from build123d import *

# Parameters (mm, degrees)
SKETCH1_R           = 25.4
BOSS_EXTRUDE1_DEPTH = 10.16
FILLET1_R           = 0.762
CUT_EXTRUDE1_DEPTH  = 11.16


with BuildPart() as part:
    # Sketch1 → Boss-Extrude1 (new body)
    with BuildSketch(Plane(origin=(0, 0, 0), x_dir=(0, 0, -1), z_dir=(1, 0, 0))):
        Circle(SKETCH1_R)
    extrude(amount=BOSS_EXTRUDE1_DEPTH)

    # Fillet1
    fillet1_edges = [part.edges().sort_by_distance(p)[0] for p in [
        (0, 0, 25.4),
        (10.16, 0, 25.4),
    ]]
    fillet(fillet1_edges, radius=FILLET1_R)

    # Sketch2 → Cut-Extrude1 (cut, through all)
    with BuildSketch(Plane(origin=(10.16, 0, 0), x_dir=(0, 0, -1), z_dir=(1, 0, 0))):
        with BuildLine():
            Line((-1.524, -2.032), (-1.524, 2.032))
            ThreePointArc((-1.524, 2.032), (0, 2.54), (1.524, 2.032))
            Line((1.524, 2.032), (1.524, -2.032))
            ThreePointArc((1.524, -2.032), (0, -2.54), (-1.524, -2.032))
        make_face()
    extrude(amount=-CUT_EXTRUDE1_DEPTH, mode=Mode.SUBTRACT)


solid = part.part
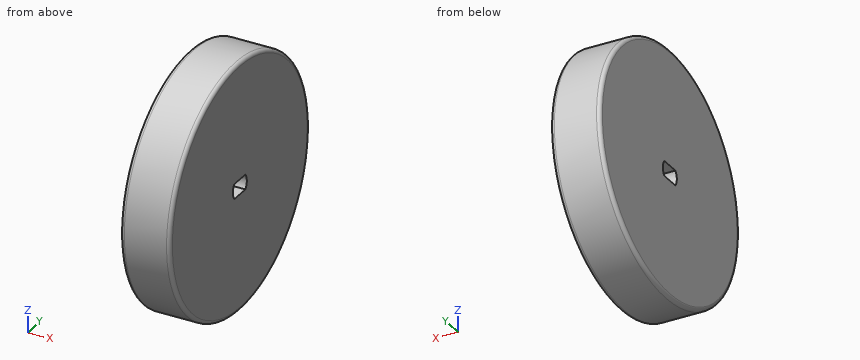
Build history of the part. All positions in model axes, mm. Coordinates: 2 decimals unless noted, no trailing zeros. Write each loop counter-clockwise with the first axis right and the second up, starting at its lowest first coordinate (ties: lowest second). Pieces come first, ordered by that corner, then holes.
(1) Cut at B-B on z = 0. List the corners of the cut face in (x, y), and give its area (3 significant figures).
(2) Cut at A-A on y = 0. List the corners of the cut face in (x, z).
(3) Pin check, flat tips, straight feed: pin 1 Ø1 at (x, y) = (4.5, 9.5) entering from +Z; pin 2 Ø4 at (x, y) = (9, 15) entering from +Z. Stop position of each tip, or through.
(4) Cut at C-C on x = 2.75. List the corners of the cut face in (y, z), and give its area (3 significant figures).
(5) Drill centre lines: line 1 (Z direction, x = 1, y = 0.5); line 2 (Z direction, x = 5.75, y = 2); line 3 (Y direction, x = 4.25, z = -17). Where is each one in solid material? Low to high.
Working result:
1. outline: (0, -24.64) arc R0.76 ccw to (0.76, -25.4) - (9.4, -25.4) arc R0.76 ccw to (10.16, -24.64) - (10.16, -2.54) - (0, -2.54) - close; (0, 2.54) - (10.16, 2.54) - (10.16, 24.64) arc R0.76 ccw to (9.4, 25.4) - (0.76, 25.4) arc R0.76 ccw to (0, 24.64) - close
1. area: 464 mm2
2. outline: (0, -24.64) arc R0.76 ccw to (0.76, -25.4) - (9.4, -25.4) arc R0.76 ccw to (10.16, -24.64) - (10.16, -1.52) - (0, -1.52) - close; (0, 1.52) - (10.16, 1.52) - (10.16, 24.64) arc R0.76 ccw to (9.4, 25.4) - (0.76, 25.4) arc R0.76 ccw to (0, 24.64) - close
3. pin 1: stops at z = 23.75
3. pin 2: stops at z = 21.82
4. outline: circle Ø50.8 at (0, 0); hole (-2.03, -1.52) - (2.03, -1.52) arc R2.54 ccw to (2.03, 1.52) - (-2.03, 1.52) arc R2.54 ccw to start
4. area: 2,010 mm2
5. line 1: z = -25.4 to -1.52, 1.52 to 25.4
5. line 2: z = -25.32 to -1.52, 1.52 to 25.32
5. line 3: y = -18.87 to 18.87
